For this review, use the dimensioned drawing (mm, ordinates from the lowest corner) and the shaded views. A direction names the side the tool comes from. Give positions to 0.01 mm unless a question says otherwise; leave off trailing zeros. Write each loop counter-clockwise with the first axis right and the second up, starting at its lowest first coordinate (ties: lowest second). Pieces come first, ordered by that corner, then holes. Notation, with made-up numbers: M -1.75,-20 L 46.25,-20 A7 cw 46.25,-15 Z; hole C -6,15.25 d7. An arc over 180 degrees is marked long. Answer in a Markdown table with one row per item.
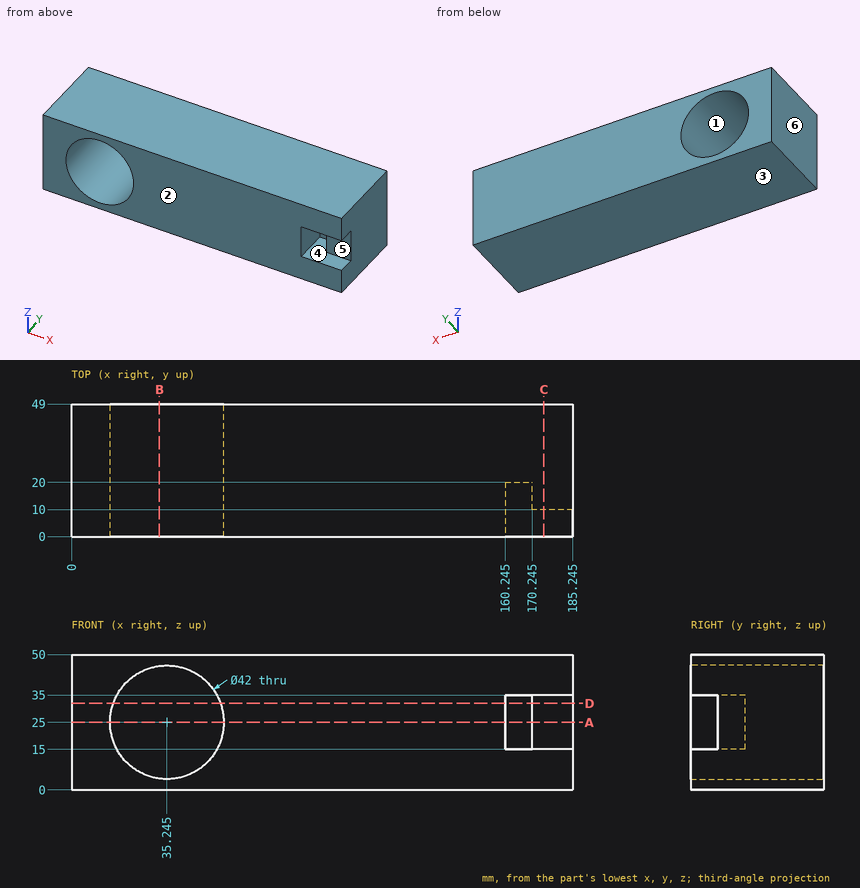
1) The part is to be moulded in two halves that separate along Z. For the marked faces 1, 2 and 3, say which applies: released by +Z, released by -Z, zero draft, split by the parting line, or undercut.
Geometry says:
| item | result |
|---|---|
| face 1 | undercut |
| face 2 | zero draft |
| face 3 | released by -Z |
2) Add section A-A (z = 25). Write out the cut boundary in (x, y) (1 decimal), and give its area (3 significant figures).
Geometry says:
| item | result |
|---|---|
| outline | M 0,0 L 14.2,0 L 14.2,49 L 0,49 Z; M 56.2,0 L 160.2,0 L 160.2,20 L 170.2,20 L 170.2,10 L 185.2,10 L 185.2,49 L 56.2,49 Z |
| area | 6,670 mm^2 |
3) Add section D-D (z = 32). Write out the cut boundary in (x, y) (1 decimal), and give its area (3 significant figures).
Geometry says:
| item | result |
|---|---|
| outline | M 0,0 L 15.4,0 L 15.4,49 L 0,49 Z; M 55,0 L 160.2,0 L 160.2,20 L 170.2,20 L 170.2,10 L 185.2,10 L 185.2,49 L 55,49 Z |
| area | 6,790 mm^2 |
4) Insertion check: P1, Ø5, axis at x = 165, z = 29.5, coming from the -Y side; P2, Ø7.5, axis at x = 179.5, z = 25, coming from the -Y side. Each pin has a flat end and moves straight along its axis. Give the tip position at first contact, or say it passes through.
Geometry says:
| item | result |
|---|---|
| P1 | y = 20 |
| P2 | y = 10 |
5) Add section B-B (x = 32.5). Write out the cut boundary in (y, z).
Geometry says:
| item | result |
|---|---|
| outline | M 0,0 L 49,0 L 49,4.18 L 0,4.18 Z; M 0,45.82 L 49,45.82 L 49,50 L 0,50 Z |
6) To check wall thickness, follow probe 1 along X at (y, z) = (12.5, 25) (1 decimal); probe 2 along X at (y, z) = (32, 25) (1 decimal); probe 3 along Z at (x, y) = (34, 32). State the ranges of each line that lie inside material, in increasing order. Write a range as [from, to].
Geometry says:
| item | result |
|---|---|
| probe 1 | [0, 14.2], [56.2, 160.2], [170.2, 185.2] |
| probe 2 | [0, 14.2], [56.2, 185.2] |
| probe 3 | [0, 4.04], [45.96, 50] |
7) For the marked faces 4, 5 and 6, list the 3-axis set-ups (+Z, -Z, +X, -X, +Y, -Y) from which the entire face can be reached by the end or side of a thin tool; tool diameter is ignored.
Geometry says:
| item | result |
|---|---|
| face 4 | -Y |
| face 5 | +X, -Y |
| face 6 | +Z, -Z, -X, +Y, -Y |
8) Add section C-C (x = 174.5). Write out the cut boundary in (y, z).
Geometry says:
| item | result |
|---|---|
| outline | M 0,0 L 49,0 L 49,50 L 0,50 L 0,35 L 10,35 L 10,15 L 0,15 Z |
